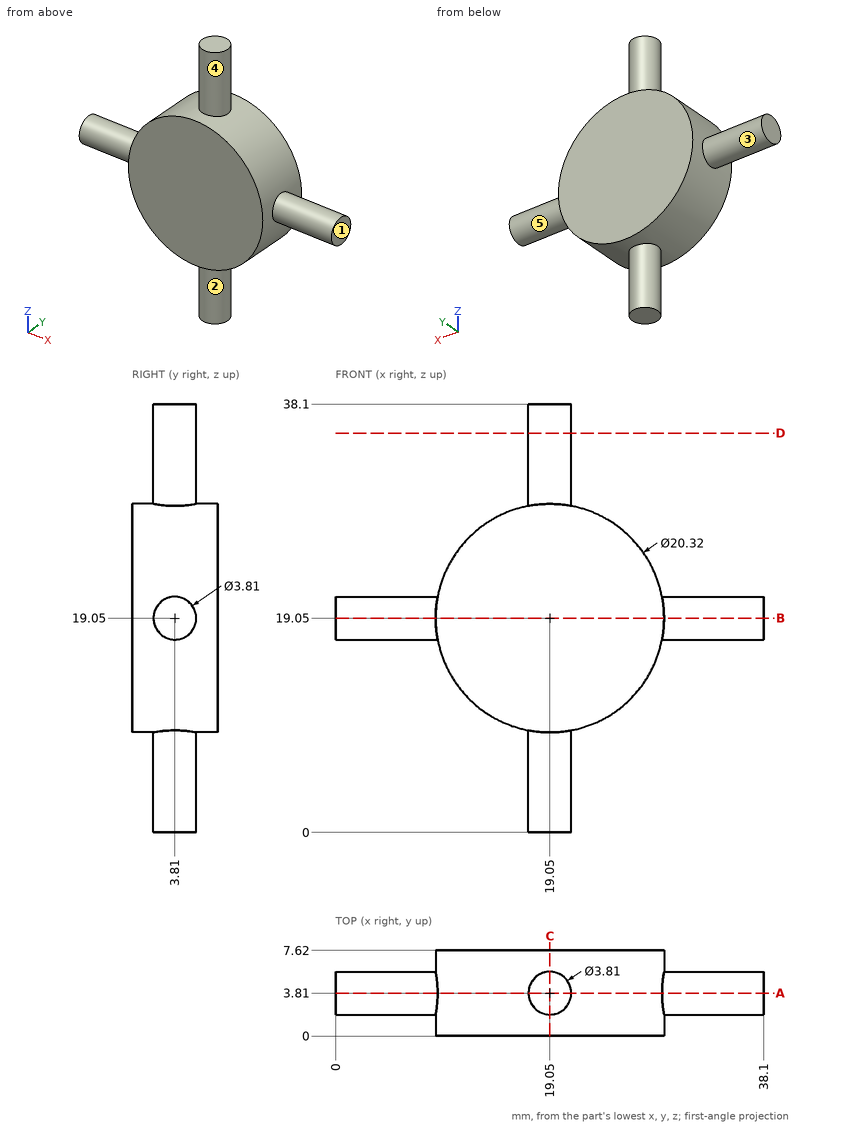
Part print with two shaded views. Sizes in mm from the minimum x, y, z corner. A direction names the side the tool comes from. Give positions to 0.01 mm unless a question says otherwise; leave off trailing zeros. Order: outer loops, then holes, each group sorted by start corner. A loop starts at its lowest first (then second) coordinate and runs counter-clockwise, first axis right, second up.
1) Saw through at B-B, the plane z = 19.05. Write the cut outline in (x, y) (3 decimals).
2) 3-axis set-ups, long thin cutter, end or side, ignore diameter. For the marked faces 1, 2, 3, 4 and 5: which of +Z, -Z, +X, -X, +Y, -Y reach the whole face in a straight line?
3) Wall check: probe 1 along Z at (x, y) = (36.5, 3); probe 2 along Z at (x, y) = (22, 7.25); probe 3 along X at (y, z) = (0.5, 19.5). Give the ranges that are in metal, low to high.
4) Saw through at D-D, the plane z = 35.5. Write the cut outline in (x, y) (3 decimals).
5) Saw through at C-C, the plane x = 19.05. Write the cut outline in (y, z) (3 decimals), then the cut area to 3 significant figures.
6) Pin check, flat tips, straight feed: pin 1 (8 mm diameter, centred on x = 4, z = 15.5, fed in from +Y) (3 decimals); pin 2 (2 mm diameter, centred on y = 3.5, z = 24, fed in from -X). Stop position of each tip, or through.
7) Saw through at A-A, the plane y = 3.81. Write the cut outline in (x, z) (3 decimals), then the cut area to 3 significant figures.
Computed:
1. outline: (0, 1.905) - (8.89, 1.905) - (8.89, 0) - (29.21, 0) - (29.21, 1.905) - (38.1, 1.905) - (38.1, 5.715) - (29.21, 5.715) - (29.21, 7.62) - (8.89, 7.62) - (8.89, 5.715) - (0, 5.715) - close
2. face 1: +Z, -Z, +X, +Y, -Y
2. face 2: -Z
2. face 3: -X
2. face 4: +Z
2. face 5: +X
3. probe 1: z = 17.33 to 20.77
3. probe 2: z = 9.33 to 28.77
3. probe 3: x = 8.9 to 29.2
4. outline: circle Ø3.81 at (19.05, 3.81)
5. outline: (0, 8.89) - (1.905, 8.89) - (1.905, 0) - (5.715, 0) - (5.715, 8.89) - (7.62, 8.89) - (7.62, 29.21) - (5.715, 29.21) - (5.715, 38.1) - (1.905, 38.1) - (1.905, 29.21) - (0, 29.21) - close
5. area: 223 mm2
6. pin 1: stops at y = 5.715
6. pin 2: stops at x = 9.69
7. outline: (0, 17.145) - (9.07, 17.145) arc R10.16 ccw to (17.145, 9.07) - (17.145, 0) - (20.955, 0) - (20.955, 9.07) arc R10.16 ccw to (29.03, 17.145) - (38.1, 17.145) - (38.1, 20.955) - (29.03, 20.955) arc R10.16 ccw to (20.955, 29.03) - (20.955, 38.1) - (17.145, 38.1) - (17.145, 29.03) arc R10.16 ccw to (9.07, 20.955) - (0, 20.955) - close
7. area: 461 mm2
